Source: CAD feature listing. Evaluate the final solid. Frame: model axes, mm. Face numbers are marked on the shaded views. Coordinates: 2 decimals unless noted, no trailing zeros. Write each loop counter-clockwise with the first axis right and the second up, starting at its lowest first coordinate (ties: lowest second). Pieces come first, ordered by that corner, then holes. Notation, with made-up numbers: M -27,39.5 L 10,39.5 A11 ccw 10,60.5 Z; hole C -1,84.5 d2. An arc over 180 degrees is marked long. One line per item, written item: value. Start each with the question number.
Item 1: Pin query (flat end, axial travel): P1, Ø1.6, axis at x = -14.05, z = 12.35, coming from the -Y side; P2, Ø3, axis at x = 14.05, z = -7.35, coming from the +Y side; P3, Ø6, axis at x = 8, y = 20.5, coming from the +Z side; P4, Ø12, axis at y = 47, z = 27.5, coming from the -X side. Return the tip coordinate at first contact, or that it passes through.
Item 2: Cut plane B-B, the plane z = -37. Output: boundary loops of the cut face in (x, y).
Item 3: Ray query, L1, parallel to X at y = -2, z = 6.5; L2, parallel to Z at x = -19.05, y = -1.2; L3, parallel to X at y = -1, z = 12. Return the intervals inside material, ascending. Write a range as from..to.
Item 4: Cut plane C-C, the plane y = 50. Output: boundary loops of the cut face in (x, z) (3 decimals).
Item 5: Cut plane A-A, the plane x = 0. Output: boundary loops of the cut face in (y, z) (3 decimals), then the cut area to 3 significant figures.
Item 6: Mould query, pull axis Z, two halves, no side actions, for the marked faces 1, 2 and 3. Classes: released by +Z, released by -Z, zero draft, split by the parting line, or undercut.
```python
from build123d import *

# Parameters (mm, degrees)
SKETCH1_R               = 51.0286
SKETCH1_R_2             = 45.085
BOSS_EXTRUDE1_DEPTH     = 57.15
SKETCH2_R               = 51.0286
BOSS_EXTRUDE2_DEPTH     = 5.08
SKETCH3_R               = 1
CUT_EXTRUDE1_DEPTH      = 1
CUT_EXTRUDE1_DEPTH_BACK = 63.23


with BuildPart() as part:
    # Sketch1 → Boss-Extrude1 (new body)
    with BuildSketch(Plane(origin=(0, 0, 0), x_dir=(1, 0, 0), z_dir=(0, 1, 0))):
        Circle(SKETCH1_R)
        Circle(SKETCH1_R_2, mode=Mode.SUBTRACT)
    extrude(amount=BOSS_EXTRUDE1_DEPTH)

    # Sketch2 → Boss-Extrude2 (add)
    with BuildSketch(Plane.XZ):
        Circle(SKETCH2_R)
    extrude(amount=BOSS_EXTRUDE2_DEPTH)

    # Sketch3 → Cut-Extrude1 (cut, two sides)
    with BuildSketch(Plane(origin=(0, -5.08, 0), x_dir=(-1, 0, 0), z_dir=(0, -1, 0))) as cut_extrude1_sk:
        with Locations((14.049999967, -7.349999968)):
            Circle(SKETCH3_R)
        with Locations((14.049999967, -12.349999968)):
            Circle(SKETCH3_R)
        with Locations((19.049999967, -12.349999968)):
            Circle(SKETCH3_R)
        with Locations((19.049999967, -7.349999968)):
            Circle(SKETCH3_R)
        with Locations((19.049999967, 7.350000032)):
            Circle(SKETCH3_R)
        with Locations((19.049999967, 12.350000032)):
            Circle(SKETCH3_R)
        with Locations((14.049999967, 12.350000032)):
            Circle(SKETCH3_R)
        with Locations((-14.050000033, 12.350000032)):
            Circle(SKETCH3_R)
        with Locations((-14.050000033, 7.350000032)):
            Circle(SKETCH3_R)
        with Locations((-19.050000033, 12.350000032)):
            Circle(SKETCH3_R)
        with Locations((-19.050000033, 7.350000032)):
            Circle(SKETCH3_R)
        with Locations((-19.050000033, -7.349999968)):
            Circle(SKETCH3_R)
        with Locations((-14.050000033, -7.349999968)):
            Circle(SKETCH3_R)
        with Locations((-14.050000033, -12.349999968)):
            Circle(SKETCH3_R)
        with Locations((-19.050000033, -12.349999968)):
            Circle(SKETCH3_R)
        with Locations((14.049999967, 7.350000032)):
            Circle(SKETCH3_R)
    extrude(amount=CUT_EXTRUDE1_DEPTH, mode=Mode.SUBTRACT)
    extrude(cut_extrude1_sk.sketch, amount=-CUT_EXTRUDE1_DEPTH_BACK, mode=Mode.SUBTRACT)


solid = part.part
```
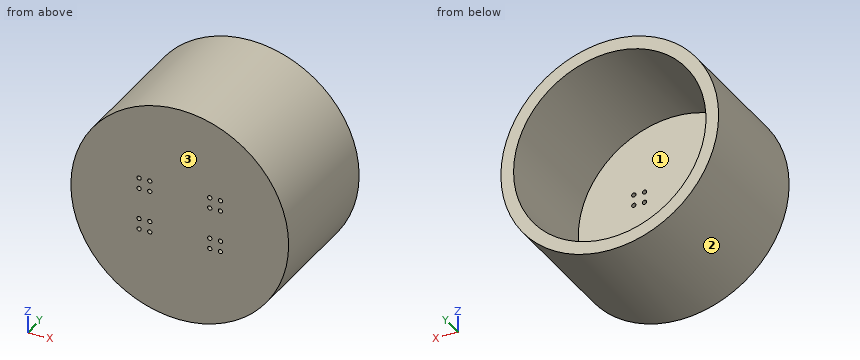
From the geometry:
1. P1: passes through
1. P2: stops at y = 0
1. P3: stops at z = 50.78
1. P4: stops at x = -46.28
2. outline: M -35.14,-5.08 L 35.14,-5.08 L 35.14,57.15 L 25.76,57.15 L 25.76,0 L -25.76,0 L -25.76,57.15 L -35.14,57.15 Z
3. L1: x = -50.61..-19.58, -18.52..-14.58, -13.52..13.52, 14.58..18.52, 19.58..50.61
3. L2: z = -47.34..-13.35, -11.35..-8.35, -6.35..6.35, 8.35..11.35, 13.35..47.34
3. L3: x = -49.6..-19.99, -18.11..-14.99, -13.11..13.11, 14.99..18.11, 19.99..49.6
4. outline: C 0,0 d102.057; hole C 0,0 d90.17
5. outline: M -5.08,-51.029 L 57.15,-51.029 L 57.15,-45.085 L 0,-45.085 L 0,45.085 L 57.15,45.085 L 57.15,51.029 L -5.08,51.029 Z
5. area: 1,200 mm²
6. face 1: undercut
6. face 2: split by the parting line
6. face 3: zero draft
